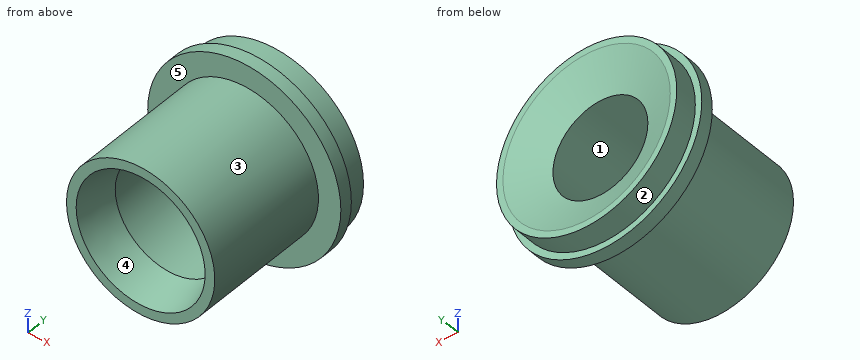
Autodesk Inventor part; units mm, degrees
ref_plane "YZ Plane" through (0, 0, 0) normal (1, 0, 0) x (0, 1, 0)
ref_plane "XZ Plane" through (0, 0, 0) normal (0, 1, 0) x (-1, 0, 0)
ref_plane "XY Plane" through (0, 0, 0) normal (0, 0, 1) x (1, 0, 0)
sketch "Sketch1" plane through (0, 0, 0) normal (0, 0, 1) x (1, 0, 0)
  line L0 (0, 25.4) -> (-28.702, 25.4) construction
  line L1 (0, 25.4) -> (-95.25, 25.4) construction
  line L2 (-95.25, 25.4) -> (-88.9, 25.4) construction
  line L3 (-88.9, 25.4) -> (-82.55, 22.4389) construction
  line L4 (-88.9, 25.4) -> (-88.9, 22.4389) construction
  line L5 (-88.9, 0) -> (-95.25, 0)
  line L6 (-28.702, 59.6457) -> (-28.702, -91.9304) construction
  arc A0 (-28.9184, -8.3597) -> (-32.3684, -0.9611) centre (-35.052, -6.7162) ccw
  line L7 (-76.2, -184.8171) -> (-28.9184, -8.3597)
  line L8 (-88.9, 22.4389) -> (-82.55, 22.4389)
  line L9 (-88.9, 22.4389) -> (-88.9, 0)
  line L10 (-82.55, 22.4389) -> (-32.3684, -0.9611)
  line L11 (-28.702, -6.7162) -> (-60.452, -6.7162) construction
  line L12 (-60.452, 12.1345) -> (-60.452, -126.0448) construction
  line L13 (-60.452, -126.0448) -> (-54.102, -126.0448) construction
  line L14 (-54.102, -126.0448) -> (-54.102, -102.3463) construction
  line L15 (-54.102, -102.3463) -> (-60.452, -102.3463)
  line L16 (-60.452, 12.1345) -> (-60.452, 2.6095) construction
  line L17 (-60.452, 12.1345) -> (-60.452, 5.7845) construction
  line L18 (-60.452, 5.7845) -> (-46.8344, 5.7845)
  line L19 (-60.452, 5.7845) -> (-60.452, -102.3463)
  line L20 (-95.25, 0) -> (-95.25, -12.7) construction
  line L21 (-60.452, -12.7) -> (-73.152, -12.7) construction
  line L22 (-95.25, -12.7) -> (-95.25, -25.4) construction
  line L23 (-95.25, -25.4) -> (-95.25, -88.9) construction
  line L24 (-95.25, -88.9) -> (-82.55, -88.9) construction
  line L25 (-82.55, -88.9) -> (-82.55, -25.4) construction
  line L26 (-95.25, -25.4) -> (-82.55, -25.4)
  line L27 (-82.55, -25.4) -> (-82.55, -88.9)
  line L28 (-82.55, -88.9) -> (-95.25, -88.9)
  line L29 (-95.25, -12.7) -> (-73.152, -12.7)
  line L30 (-73.152, -137.8941) -> (-63.627, -137.8941)
  line L31 (-82.55, -88.9) -> (-82.55, -184.8171)
  line L32 (-82.55, -184.8171) -> (-76.2, -184.8171)
  line L33 (-73.152, -12.7) -> (-73.152, -137.8941)
  line L34 (-88.9, -25.4) -> (-88.9, -31.3436)
  line L35 (-88.9, -31.3436) -> (-95.25, -31.3436)
  line L36 (-95.25, 0) -> (-95.25, -25.4)
  line L37 (-95.25, -31.3436) -> (-95.25, -88.9)
  line L38 (0, -319.0244) -> (0, 122.7573)
  point P0 (0, 0)
  point P1 (-95.25, -255.9127)
  point P2 (-85.725, 22.4389)
  dimension "d0" = 28.702
  dimension "d1" = 95.25
  dimension "d2" = 6.35
  dimension "d3" = 25
  dimension "d5" = 25.4
  dimension "d6" = 25.4
  dimension "d8" = 12.7
  dimension "d11" = 6.35
  dimension "d12" = 31.75
  dimension "d13" = 6.35
  dimension "d15" = 6.35
  dimension "d16" = 12.7
  dimension "d17" = 12.7
  dimension "d18" = 12.7
  dimension "d19" = 63.5
  dimension "d20" = 12.7
  dimension "d22" = 9.525
  dimension "d23" = 6.35
  dimension "d25" = 5.9436
  dimension "d26" = 15
revolve "Revolution2" add sketch "Sketch1" angle 360 about axis through (0, -10, 0) along (0, 1, 0) contours L9 L8 L10 L18 L19 L15 L7 L30 L33 L29 L36 L5
properties part number "Phenolic Master Sketch" material "Phenolic Resin"
Geometry check sheet. Reference: the model listing, model coordinates, mm. Face numbers are marked on the shaded views. A direction names the side the tool comes from. Round coordinates to 2 decimals unless told otherwise and drop trailing zeros. Write each loop counter-clockwise with the first axis right and the second up, starting at its lowest first coordinate (ties: lowest second). Pieces come first, ordered by that corner, then holes.
Item 1: Section check C-C (y = -89.5). Record the boundary of the cut face in (x, z), plus the area to 3 significant figures.
Determined:
outline: circle Ø146.3 at (0, 0); hole circle Ø120.9 at (0, 0)
area: 5,330 mm2
Item 2: Section check A-A (x = 0). Record the boundary of the cut face in (y, z), plus the area to 3 significant figures.
Determined:
outline: (-137.89, -73.15) - (-12.7, -73.15) - (-12.7, -95.25) - (0, -95.25) - (0, -88.9) - (22.44, -88.9) - (22.44, -82.55) - (5.78, -46.83) - (5.78, -60.45) - (-102.35, -60.45) - (-102.35, -54.1) - (-137.89, -63.63) - close; (-137.89, 63.63) - (-102.35, 54.1) - (-102.35, 60.45) - (5.78, 60.45) - (5.78, 46.83) - (22.44, 82.55) - (22.44, 88.9) - (0, 88.9) - (0, 95.25) - (-12.7, 95.25) - (-12.7, 73.15) - (-137.89, 73.15) - close
area: 5,310 mm2
Item 3: Go/stop test with flat-tipped pins: pin 1 Ø3 at (x, y) = (11, -90) entering from +Z; pin 2 Ø2 at (y, z) = (-94, -43) entering from +X; pin 3 Ø5 at (x, z) = (40, -14) entering from +Y; pin 4 Ø3 at (x, y) = (-38.5, -1) entering from -Z. Record where each tip stops, or that it passes through.
Determined:
pin 1: stops at z = 72.53
pin 2: stops at x = 59.89
pin 3: passes through
pin 4: stops at z = -87.77
Item 4: Section check D-D (y = -116). Record the boundary of the cut face in (x, z), plus the area to 3 significant figures.
Determined:
outline: circle Ø146.3 at (0, 0); hole circle Ø115.52 at (0, 0)
area: 6,330 mm2
Item 5: Material ranges on line 1 along Z through (x, y) = (0, -30.5); line 2 along Z through (x, y) = (-48, -117.5); line 3 along X through (y, z) = (-13, 11.5), recorded low to high.
Determined:
line 1: z = -73.15 to -60.45, 60.45 to 73.15
line 2: z = -55.2 to -32.85, 32.85 to 55.2
line 3: x = -72.24 to -59.35, 59.35 to 72.24
Item 6: Access from +Z, -Z, +X, -X, +Y, -Y to the whole of each face (thin tool, end or side, straight path). Record for the marked faces 1 and 2.
Determined:
face 1: none
face 2: +Y
Item 7: Section check B-B (z = 0). Record the boundary of the cut face in (x, y).
Determined:
outline: (-95.25, -12.7) - (-73.15, -12.7) - (-73.15, -137.89) - (-63.63, -137.89) - (-54.1, -102.35) - (-60.45, -102.35) - (-60.45, 5.78) - (-46.83, 5.78) - (-82.55, 22.44) - (-88.9, 22.44) - (-88.9, 0) - (-95.25, 0) - close; (46.83, 5.78) - (60.45, 5.78) - (60.45, -102.35) - (54.1, -102.35) - (63.63, -137.89) - (73.15, -137.89) - (73.15, -12.7) - (95.25, -12.7) - (95.25, 0) - (88.9, 0) - (88.9, 22.44) - (82.55, 22.44) - close
Item 8: Mould release check, pull along Z, two halves, no side actions. Record for the marked faces 3, 4 and 5: +Z half, -Z half, draft (parallel to the pull), parting line (faces both ways), or undercut.
Determined:
face 3: parting line
face 4: undercut
face 5: draft
